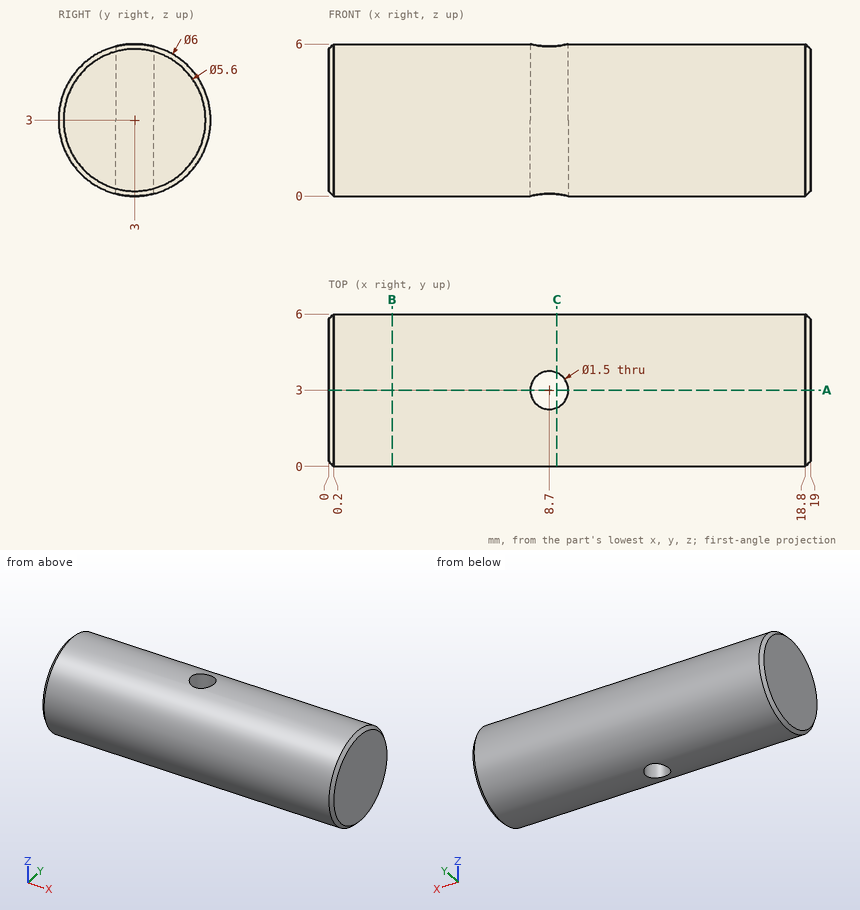
Study the drawing (mm; zero at the part's minimum x, y, z) and answer. Round coordinates to 2 decimals unless told otherwise and drop trailing zeros. Write each loop counter-clockwise with the first axis right and the second up, starting at its lowest first coordinate (ties: lowest second). Pieces come first, ordered by that corner, then holes.
1) Flat-ended cylindrical pins translate along their axes: P1, Ø3, axis at x = 11.5, y = 5, coming from the +Z side; P2, Ø3, axis at x = 7.5, y = 1, coming from the -Z side. Find the tip coordinate at first contact, or state that the pin passes through.
2) A cutting plane is placed at A-A on y = 3. Determine the outline of the cut face in (x, z).
3) A cutting plane is placed at B-B on x = 2.5. Determine the outline of the cut face in (y, z).
4) Consider probe 1 along Y at (x, z) = (8.7, 1.95); probe 2 along Y at (x, z) = (8.7, 4.2); probe 3 along X at (y, z) = (3.25, 2.5). Determine where each line is inside the solid, lowest interval first.
5) A cutting plane is placed at C-C on x = 9. Determine the outline of the cut face in (y, z), and give its area (3 significant figures).
Entries:
1. P1: stops at z = 5.96
1. P2: stops at z = 0.04
2. outline: (0, 0.2) - (0.2, 0) - (7.95, 0) - (7.95, 6) - (0.2, 6) - (0, 5.8) - close; (9.45, 0) - (18.8, 0) - (19, 0.2) - (19, 5.8) - (18.8, 6) - (9.45, 6) - close
3. outline: circle Ø6 at (3, 3)
4. probe 1: y = 0.19 to 2.25, 3.75 to 5.81
4. probe 2: y = 0.25 to 2.25, 3.75 to 5.75
4. probe 3: x = 0 to 7.99, 9.41 to 19
5. outline: (2.31, 0.08) - (2.31, 5.92) arc R3 ccw to start; (3.69, 0.08) arc R3 ccw to (3.69, 5.92) - close
5. area: 20.1 mm2
